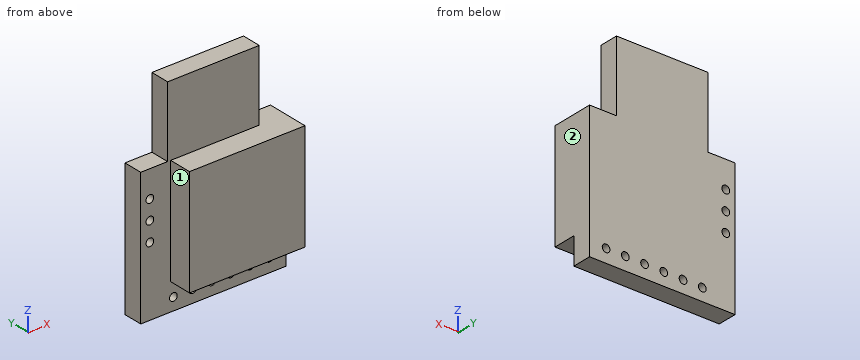
```python
from build123d import *

# Parameters (mm, degrees)
F1_DEPTH = 5.5
F0_R     = 0.5
F2_DEPTH = 2.5


with BuildPart() as f1:
    # F0 (on Front) → F1 (new body)
    with BuildSketch(Plane.XZ):
        Polygon((14.10483, 19.007904), (2.70483, 19.007904), (2.70483, 5.007904), (17.70483, 5.007904), (17.70483, 19.007904), (14.864999, 19.007904), (14.50483, 19.007904), (14.20483, 19.007904), align=None)
    extrude(amount=F1_DEPTH)

    # F0 (on Front) → F2 (join)
    with BuildSketch(Plane.XZ):
        Polygon((2.30483, 19.007904), (-1.19517, 19.007904), (-1.19517, 1.507904), (17.70483, 1.507904), (17.70483, 5.007904), (2.70483, 5.007904), (2.70483, 19.007904), align=None)
        with Locations((3.05315, 3.12218)):
            Circle(F0_R, mode=Mode.SUBTRACT)
        with Locations((5.553036, 3.146059)):
            Circle(F0_R, mode=Mode.SUBTRACT)
        with Locations((8.052922, 3.169939)):
            Circle(F0_R, mode=Mode.SUBTRACT)
        with Locations((0, 10.509157)):
            Circle(F0_R, mode=Mode.SUBTRACT)
        with Locations((0, 13.009157)):
            Circle(F0_R, mode=Mode.SUBTRACT)
        with Locations((10.552808, 3.193818)):
            Circle(F0_R, mode=Mode.SUBTRACT)
        with Locations((13.052693, 3.217697)):
            Circle(F0_R, mode=Mode.SUBTRACT)
        with Locations((15.552579, 3.241576)):
            Circle(F0_R, mode=Mode.SUBTRACT)
        with Locations((0, 15.509157)):
            Circle(F0_R, mode=Mode.SUBTRACT)
        Polygon((2.30483, 28.207904), (2.30483, 19.007904), (2.70483, 19.007904), (14.10483, 19.007904), (14.20483, 19.007904), (14.20483, 28.207904), align=None)
        Polygon((14.10483, 19.007904), (2.70483, 19.007904), (2.70483, 5.007904), (17.70483, 5.007904), (17.70483, 19.007904), (14.864999, 19.007904), (14.50483, 19.007904), (14.20483, 19.007904), align=None)
    extrude(amount=F2_DEPTH)


solid = f1.part
```
Check sheet for the modelled part. Datum: model origin and axes. Units: mm. Face numbers are marked on the shaded views. A direction names the side the tool comes from. Round coordinates to 2 decimals unless told otherwise and drop trailing zeros. Write each loop counter-clockwise with the first axis right and the second up, starting at its lowest first coordinate (ties: lowest second). Pieces come first, ordered by that corner, then holes. Notation, with made-up numbers: (4, 5) -> (37, 5) arc R29 cw to (37, 32) -> close; hole circle Ø4 at (78.25, 21). An arc over 180 degrees is marked (long way). One line per question, with ' | ' between items. Start each with the question number.
1. Set-up check for the marked faces 1 and 2: record each of +Z, -Z, +X, -X, +Y, -Y from which the full face is reachable in a straight line by a thin tool's end or side.
2. Sectioned sample at D-D, the plane x = 8. Record the cut outline in (y, z).
3. Sectioned sample at B-B, the plane z = 8.25. Record the cut outline in (x, y).
4. Sectioned sample at C-C, the plane y = -1.3. Count the separate pieces of the cut face and the enclosed holes in it, then the cut area to 3 significant figures.
5. Sectioned sample at A-A, the plane x = 0. Record the cut outline in (y, z), then the cut area to 4 significant figures.
6. Depth check by flat-ended pin: pin 1 (1.2 mm diameter, centred on x = 0.5, y = -1.5, fed in from +Z); pin 2 (8 mm diameter, centred on x = 8.5, z = 25, fed in from -Y); pin 3 (2 mm diameter, centred on y = -1.5, z = 23, fed in from -X); pin 4 (5 mm diameter, centred on x = 15.5, z = 21, fed in from -Y). Enter the tip coordinate at first touch or a pass-through.
7. Scan lines: line 1 along Z through (x, y) = (0, -1.5); line 2 along Z through (x, y) = (10.25, -4.1); line 3 along X through (y, z) = (-2.2, 23.75). Record each from-to range of solid material in increasing order. Write a range as from..to.
Taken from the geometry:
1) face 1: +Z, -Z, -X, -Y | face 2: +Z, -Z, +X, +Y, -Y
2) outline: (-5.5, 5.01) -> (-2.5, 5.01) -> (-2.5, 3.67) -> (0, 3.67) -> (0, 28.21) -> (-2.5, 28.21) -> (-2.5, 19.01) -> (-5.5, 19.01) -> close; (-2.5, 1.51) -> (0, 1.51) -> (0, 2.67) -> (-2.5, 2.67) -> close
3) outline: (-1.2, -2.5) -> (2.7, -2.5) -> (2.7, -5.5) -> (17.7, -5.5) -> (17.7, 0) -> (-1.2, 0) -> close
4) separate pieces: 1 | enclosed holes: 9 | area: 433 mm^2
5) outline: (-2.5, 1.51) -> (0, 1.51) -> (0, 10.01) -> (-2.5, 10.01) -> close; (-2.5, 11.01) -> (0, 11.01) -> (0, 12.51) -> (-2.5, 12.51) -> close; (-2.5, 13.51) -> (0, 13.51) -> (0, 15.01) -> (-2.5, 15.01) -> close; (-2.5, 16.01) -> (0, 16.01) -> (0, 19.01) -> (-2.5, 19.01) -> close | area: 36.25 mm^2
6) pin 1: stops at z = 19.01 | pin 2: stops at y = -2.5 | pin 3: stops at x = 2.3 | pin 4: stops at y = -5.5
7) line 1: z = 1.51..10.01, 11.01..12.51, 13.51..15.01, 16.01..19.01 | line 2: z = 5.01..19.01 | line 3: x = 2.3..14.2
